from build123d import *

# Parameters (mm, degrees)
SKETCH_1_R           = 1.75
EXTRUDE_1_DEPTH      = 0.8
SKETCH_2_R           = 17.5
EXTRUDE_2_DEPTH      = 13.7
SKETCH_3_R           = 5
EXTRUDE_3_DEPTH      = 1.5
SKETCH_4_R           = 1
EXTRUDE_4_DEPTH      = 6
SKETCH_6_W           = 27
SKETCH_6_H           = 10
EXTRUDE_5_DEPTH      = 0.5
EXTRUDE_5_DEPTH_BACK = 0.5
SKETCH_7_W           = 8
SKETCH_7_H           = 10
EXTRUDE_6_DEPTH      = 6


with BuildPart() as part:
    # Sketch 1 → Extrude 1 (new body)
    with BuildSketch(Plane.XY):
        with BuildLine():
            ThreePointArc((23.382857143, 2.698516599), (24.6, 0), (23.382857143, -2.698516599))
            Line((23.382857143, -2.698516599), (11.583333333, -13.117789024))
            ThreePointArc((11.583333333, -13.117789024), (0, -17.5), (-11.583333333, -13.117789024))
            Line((-11.583333333, -13.117789024), (-23.382857143, -2.698516599))
            ThreePointArc((-23.382857143, -2.698516599), (-24.6, 0), (-23.382857143, 2.698516599))
            Line((-23.382857143, 2.698516599), (-11.583333333, 13.117789024))
            ThreePointArc((-11.583333333, 13.117789024), (0, 17.5), (11.583333333, 13.117789024))
            Line((11.583333333, 13.117789024), (23.382857143, 2.698516599))
        make_face()
        with Locations((-21, 0)):
            Circle(SKETCH_1_R, mode=Mode.SUBTRACT)
        with Locations((21, 0)):
            Circle(SKETCH_1_R, mode=Mode.SUBTRACT)
    extrude(amount=EXTRUDE_1_DEPTH)

    # Sketch 2 → Extrude 2 (add)
    with BuildSketch(Plane.XY.offset(0.8)):
        Circle(SKETCH_2_R)
    extrude(amount=EXTRUDE_2_DEPTH)

    # Sketch 3 → Extrude 3 (add)
    with BuildSketch(Plane(origin=(0, 0, 0), x_dir=(-1, 0, 0), z_dir=(0, 0, -1))):
        Circle(SKETCH_3_R)
    extrude(amount=EXTRUDE_3_DEPTH)

    # Sketch 4 → Extrude 4 (add)
    with BuildSketch(Plane(origin=(0, 0, -1.5), x_dir=(-1, 0, 0), z_dir=(0, 0, -1))):
        Circle(SKETCH_4_R)
    extrude(amount=EXTRUDE_4_DEPTH)



with BuildPart() as body_2:
    # Sketch 6 → Extrude 5 (new body, two sides)
    with BuildSketch(Plane(origin=(0, 17.5, 0), x_dir=(1, 0, 0), z_dir=(0, 1, 0))) as extrude_5_sk:
        with Locations((-7.5, -9.5)):
            Rectangle(SKETCH_6_W, SKETCH_6_H)
    extrude(amount=EXTRUDE_5_DEPTH)
    extrude(extrude_5_sk.sketch, amount=-EXTRUDE_5_DEPTH_BACK)


with BuildPart() as part_1:
    add(part.part)

    add(body_2.part)  # Extrude 6 merges body 2
    # Sketch 7 → Extrude 6 (add)
    with BuildSketch(Plane.XZ.offset(-17)):
        with Locations((-17, 9.5)):
            Rectangle(SKETCH_7_W, SKETCH_7_H)
    extrude(amount=EXTRUDE_6_DEPTH)


solid = part_1.part
The listing builds one solid part. Answer for the finished solid, in the listing's coordinates (mm). A direction names the side the tool comes from. Give positions to 0.01 mm unless a question says otherwise; leave off trailing zeros. Loops run counter-clockwise (first coordinate to the right, second up) from the corner with the lowest first, then second, coordinate; pieces in that order, holes last. Notation, with made-up numbers: M 7,49 L 53,49 A19 cw 53,65 Z; hole C 19.5,-21 d5. An arc over 180 degrees is marked long. Answer as CSV lines item,"result".
Item 1: The part is cut by section D-D (x = 21). Give the vertices of the cut face in (y, z).
Values follow:
outline,"M -4.8,0 L -1.75,0 L -1.75,0.8 L -4.8,0.8 Z; M 1.75,0 L 4.8,0 L 4.8,0.8 L 1.75,0.8 Z"
Item 2: Which of the six approach directions +Z, -Z, +X, -X, +Y, -Y give full straight-line access (tool end or side, diameter ignored) to faces 1 (the flat face through (-8, 18, 9)), 2 (the cylindrical face through (0, -1, -4))?
Values follow:
face 1,"+Z, -Z, +X, -X, +Y"
face 2,"-Z"
Item 3: The part is cut by section C-C (x = 0). Give the vertices of the cut face in (y, z).
Values follow:
outline,"M -17.5,0 L -5,0 L -5,-1.5 L -1,-1.5 L -1,-7.5 L 1,-7.5 L 1,-1.5 L 5,-1.5 L 5,0 L 17.5,0 L 17.5,4.5 L 18,4.5 L 18,14.5 L -17.5,14.5 Z"
Item 4: The mould has two halves that part along X. Classify faces 3 (the flat face through (-13, 14, 9)), 4 (the flat face through (-19, 0, 0.8)), 5 (the cylindrical face through (24.6, 0, 0.4)): released by +X, released by -X, zero draft, split by the parting line, or undercut.
Values follow:
face 3,"undercut"
face 4,"zero draft"
face 5,"released by +X"
Item 5: Straight lines are drawn through the part: line 1 along Z through (x, y) = (-17, -5.5); line 2 along Z through (x, y) = (10, -1.5); line 3 along Y through (x, z) = (21, 0.4). For each, find the intervals that lie inside material, in ascending order. Write a range as [from, to].
Values follow:
line 1,"z = [0, 0.8]"
line 2,"z = [0, 14.5]"
line 3,"y = [-4.8, -1.75], [1.75, 4.8]"
Item 6: The part is cut by section B-B (z = 5.25). Give the vertices of the cut face in (x, y).
Values follow:
outline,"M -21,11 L -13.61,11 A17.5 ccw long 4.15,17 L 6,17 L 6,18 L -21,18 Z; hole M -13,11.72 A17.5 cw -4.15,17 L -13,17 Z"
Item 7: Given pin 1 Ø3 at (y, z) = (-4, 6.5) entering from -X; pin 2 Ø4 at (y, z) = (13.5, 12) entering from +X; pin 3 Ø6 at (x, z) = (11.5, -5.5) entering from -Y; pin 4 Ø4 at (x, y) = (21, 0) entering from +Z, each flat-ended and moving along its own axis, determine where each tip first touches the part or whether it passes through.
Values follow:
pin 1,"stops at x = -17.32"
pin 2,"stops at x = 13.19"
pin 3,"passes through"
pin 4,"stops at z = 0.8"
